For this review, take the finished solid that the model builds, in its own axes (mm). A direction names the side the tool comes from. Give positions to 0.01 mm unless a question says otherwise; leave off trailing zeros. Loops run counter-clockwise (first coordinate to the right, second up) from the corner with the lowest first, then second, coordinate; pieces in that order, holes last. Notation, with made-up numbers: M 24.25,54.5 L 70.25,54.5 A11 cw 70.25,71.5 Z; hole C -32,-4 d5. An arc over 180 degrees is marked long. Use CSV: the item, a comma, the result in double quotes. Start each with the question number.
1. Take a section at A-A, the plane y = -18.5. Write out the cut boundary in (x, z).
2. Take a section at C-C, the plane x = 6. Write out the cut boundary in (y, z), and give its area (3 significant figures).
3. Take a section at D-D, the plane z = 21.5. Write out the cut boundary in (x, y), and give its area (3 significant figures).
4. Tool access review of faces 1 (the face through (-8, 5, 21)), 2 (the face through (6.466, -2.681, 9.904)), 3 (the face through (13, -1, 28)), 4 (the face through (-5, -10, 22)): name each direction out of +Z, -Z, +X, -X, +Y, -Y from which nothing blocks a thin tool from reaching the whole face with its end or side.
5. Take a section at B-B, the plane z = 40. Write out the cut boundary in (x, y).
6. Insertion check: P1, Ø5, axis at x = -12, z = 21, coming from the -Y side; P2, Ø0.8, axis at x = 0, z = 51, coming from the -Y side; P3, Ø4, axis at x = -0.5, z = 12, coming from the +Y side; P4, Ø4, axis at y = -15, z = 19, coming from the +X side. Each pin has a flat end and moves straight along its axis. Give the tip position at first contact, or say it passes through.
7. To check wall thickness, follow line 1 (Y direction, x = 1.5, z = 18); line 2 (X direction, y = -3.5, z = 4.5); line 3 (Y direction, x = -1.5, z = 20). State the ranges of each line that lie inside material, in increasing order. Write a range as [from, to].
8. The part is to be moulded in two halves that separate along Z. For faces 5 (the face through (-0.07, 15.304, 23.987)), 6 (the face through (3.01, -3.01, 0)), 7 (the face through (-11.77, -26.82, 30.5)), say which applies: pulls with the +Z half, pulls with the -Z half, needs draft (parallel to the pull), parting line crosses it, or undercut.
from build123d import *

# Parameters (mm, degrees)
F0_R          = 7
F0_R_2        = 4.1
F1_DEPTH      = 50.8
F3_DEPTH      = 31
F3_DEPTH_BACK = 13
F4_D          = 8
F4_DEPTH      = 50.8
F4_TIP        = 2.4034424761
F5_R          = 5
F7_DEPTH      = 5
F9_DEPTH      = 5
F10_D         = 8.2
F10_DEPTH     = 50.8
F10_TIP       = 2.463528538


with BuildPart() as f1:
    # F0 (on Top) → F1 (new body)
    with BuildSketch(Plane.XY):
        Circle(F0_R)
        Circle(F0_R_2, mode=Mode.SUBTRACT)
    extrude(amount=F1_DEPTH)

    # F2 (on Right) → F3 (join, two sides)
    with BuildSketch(Plane.YZ) as f3_sk:
        Polygon((0, 25.5047638916), (24.8914179106, 23.3270470053), (24.8889016367, 28.5443344728), (0, 30.7218312136), align=None)
        Polygon((-26.9524334618, 27.8627962739), (0, 25.5047638916), (0, 30.7218312136), (-26.6906069858, 33.0569567475), align=None)
    extrude(amount=-F3_DEPTH)
    extrude(f3_sk.sketch, amount=F3_DEPTH_BACK)

    # F4
    with Locations(Plane(origin=(0, 0, 0), x_dir=(1, 0, 0), z_dir=(0, 0, -1))):
        with Locations((0, 0)):
            Hole(F4_D / 2, depth=F4_DEPTH)
            with Locations((0, 0, -(F4_DEPTH + F4_TIP / 2))):  # 118° drill point
                Cone(0, F4_D / 2, F4_TIP, mode=Mode.SUBTRACT)

    # F5
    f5_edges = [f1.edges().sort_by_distance(p)[0] for p in [
        (13, 24.89016, 25.935691),
        (13, -26.82152, 30.459877),
    ]]
    fillet(f5_edges, radius=F5_R)

    # F6 (on Right) → F7 (join, symmetric)
    with BuildSketch(Plane.YZ):
        Polygon((0, 9.7866365686), (18.7852662057, 23.5712174326), (0, 25.8125010878), (-21.4374996722, 27.7812518179), align=None)
        Polygon((-21.0000015795, 33.0312512815), (0, 31.0625005513), (19.4687508047, 29.3125007302), (0, 45.9375008941), align=None)
    extrude(amount=F7_DEPTH, both=True)

    # F8 (on Front) → F9 (join, symmetric)
    with BuildSketch(Plane.XZ):
        Polygon((0, 51.6971051693), (-17.865261063, 30.367417261), (0, 0), align=None)
    extrude(amount=F9_DEPTH, both=True)

    # F10
    with Locations(Plane(origin=(0, 0, 0), x_dir=(1, 0, 0), z_dir=(0, 0, -1))):
        with Locations((0, 0)):
            Hole(F10_D / 2, depth=F10_DEPTH)
            with Locations((0, 0, -(F10_DEPTH + F10_TIP / 2))):  # 118° drill point
                Cone(0, F10_D / 2, F10_TIP, mode=Mode.SUBTRACT)


solid = f1.part
Result set:
1,outline,"M -31,27.12 L -5,27.12 L -5,25.32 L 5,25.32 L 5,27.12 L 13,27.12 L 13,32.34 L -31,32.34 Z; M -5,32.8 L 5,32.8 L 5,34.57 L -5,34.57 Z"
2,outline,"M -26.95,27.86 L -3.61,25.82 L -3.61,0 L 3.61,0 L 3.61,25.19 L 24.89,23.33 L 24.89,28.54 L 3.61,30.41 L 3.61,50.8 L -3.61,50.8 L -3.61,31.04 L -26.69,33.06 Z"
2,area,"598 mm2"
3,outline,"M -12.65,-5 L -5,-5 L -5,-13.95 L 5,-13.95 L 5,-4.9 A7 ccw 5,4.9 L 5,15.96 L -5,15.96 L -5,5 L -12.65,5 Z; hole C 0,0 d8.2"
3,area,"336 mm2"
4,face 1,"-Z, -X"
4,face 2,"-Z"
4,face 3,"+Z, -Z, +X, +Y, -Y"
4,face 4,"-Z, -X, -Y"
5,outline,"M -9.8,-5 L -5,-5 L -5,-9.66 L 5,-9.66 L 5,-4.9 A7 ccw 5,4.9 L 5,6.95 L 0.81,6.95 A7 ccw -0.81,6.95 L -5,6.95 L -5,5 L -9.8,5 Z; hole C 0,0 d8.2"
6,P1,"y = -5"
6,P2,"y = -7"
6,P3,"y = 7"
6,P4,"through"
7,line 1,"[-9.78, -3.82], [3.82, 11.19]"
7,line 2,"[-6.06, -2.14], [2.14, 6.06]"
7,line 3,"[-12.17, -3.82], [3.82, 13.92]"
8,face 5,"undercut"
8,face 6,"pulls with the -Z half"
8,face 7,"pulls with the +Z half"
